Read the model definition and answer for the solid it produces. Units are mm, in the model's axes. Face numbers are marked on the shaded views. A direction names the side the tool comes from. Give positions to 0.01 mm unless a question says otherwise; leave off trailing zeros. Order: outer loops, then holes, each group sorted by start corner. A loop starts at its lowest first (then second) coordinate and runs counter-clockwise, first axis right, second up. Notation, with made-up numbers: (0.25, 43) -> (35.25, 43) arc R17 ccw to (35.25, 55) -> close; hole circle Ø7 at (79.25, 52). An arc over 180 degrees is marked (long way). One line per question, with ' | ' between items. Start each with the question number.
```python
from build123d import *

# Parameters (mm, degrees)
BASE_FLANGE1_DEPTH = 52
CUT_EXTRUDE1_DEPTH = 88.177978871
FILLET1_R          = 2
SKETCH7_R          = 12
SKETCH7_R_2        = 1.75
CUT_EXTRUDE2_DEPTH = 10
SKETCH8_R          = 2.8
CUT_EXTRUDE3_DEPTH = 2
SKETCH9_W          = 8
SKETCH9_H          = 10
CUT_EXTRUDE4_DEPTH = 10
SKETCH10_R         = 2.1
CUT_EXTRUDE5_DEPTH = 10


# Sheet-metal steps are written as plain solids
with BuildPart() as part:
    # Sketch1 → Base-Flange1 (new body)
    with BuildSketch(Plane(origin=(0, 0, 0), x_dir=(1, 0, 0), z_dir=(0, 1, 0))):
        with BuildLine():
            Line((36, 0), (2.8, 0))
            ThreePointArc((2.8, 0), (0.820101013, 0.820101013), (0, 2.8))
            Line((0, 2.8), (0, 60))
            Line((0, 60), (2, 60))
            Line((2, 60), (2, 2.8))
            ThreePointArc((2, 2.8), (2.234314575, 2.234314575), (2.8, 2))
            Line((2.8, 2), (36, 2))
            Line((36, 2), (36, 0))
        make_face()
    extrude(amount=BASE_FLANGE1_DEPTH)

    # Sketch6 → Cut-Extrude1 (cut, through all)
    with BuildSketch(Plane.ZY):
        Polygon((-18.8, 52), (-2.8, 36), (0, 36), (0, 52), align=None)
        Polygon((-60, 52), (-58.585786438, 52), (-60, 50.585786438), align=None)
        Polygon((-60, 1.414213562), (-60, 0), (-58.585786438, 0), align=None)
    extrude(amount=-CUT_EXTRUDE1_DEPTH, mode=Mode.SUBTRACT)

    # Fillet1
    fillet1_edges = [part.edges().sort_by_distance(p)[0] for p in [
        (36, 36, -1),
        (36, 0, -1),
    ]]
    fillet(fillet1_edges, radius=FILLET1_R)

    # Sketch7 → Cut-Extrude2 (cut)
    with BuildSketch(Plane(origin=(2, 0, 0), x_dir=(0, 0, -1), z_dir=(1, 0, 0))):
        with Locations((39, 31)):
            Circle(SKETCH7_R)
        with Locations((54.5, 46.5)):
            Circle(SKETCH7_R_2)
        with Locations(Location((23.5, 46.5, 0), (0, 0, 180))):
            Circle(SKETCH7_R_2)
        with Locations(Location((54.5, 15.5, 0), (0, 0, 180))):
            Circle(SKETCH7_R_2)
        with Locations((23.5, 15.5)):
            Circle(SKETCH7_R_2)
    extrude(amount=-CUT_EXTRUDE2_DEPTH, mode=Mode.SUBTRACT)

    # Sketch8 → Cut-Extrude3 (cut)
    with BuildSketch(Plane.XY):
        with Locations((28, 29)):
            Circle(SKETCH8_R)
        with Locations(Location((28, 9, 0), (0, 0, 180))):
            Circle(SKETCH8_R)
        with Locations((8, 9)):
            Circle(SKETCH8_R)
        with Locations(Location((8, 29, 0), (0, 0, 180))):
            Circle(SKETCH8_R)
    extrude(amount=-CUT_EXTRUDE3_DEPTH, mode=Mode.SUBTRACT)

    # Sketch9 → Cut-Extrude4 (cut)
    with BuildSketch(Plane(origin=(0, 0, -2), x_dir=(-1, 0, 0), z_dir=(0, 0, -1))):
        with Locations((-18, 27)):
            Rectangle(SKETCH9_W, SKETCH9_H)
    extrude(amount=-CUT_EXTRUDE4_DEPTH, mode=Mode.SUBTRACT)

    # Sketch10 → Cut-Extrude5 (cut)
    with BuildSketch(Plane(origin=(2, 0, 0), x_dir=(0, 0, -1), z_dir=(1, 0, 0))):
        with Locations((15, 34)):
            Circle(SKETCH10_R)
    extrude(amount=-CUT_EXTRUDE5_DEPTH, mode=Mode.SUBTRACT)


solid = part.part
```
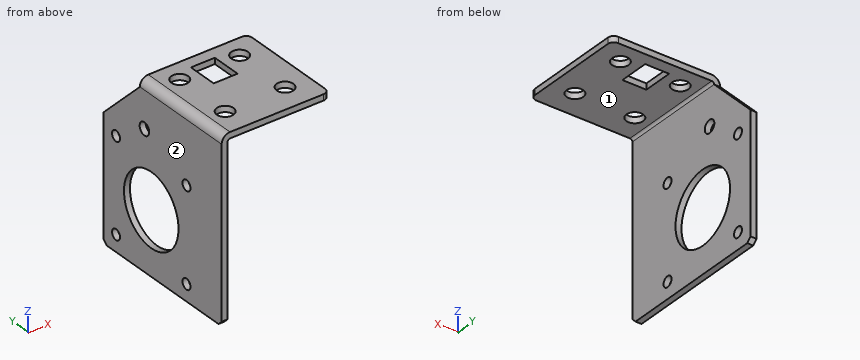
Q1. A cutting plane is placed at A-A, the plane z = -15. Determine the outline of the cut face in (x, y), then the cut area to 3 significant figures.
Q2. Find the intervals of material crossed by line 1 (Y direction, x = 8, z = -1.3); line 2 (Y direction, x = 1.15, z = -23.5); line 3 (Z direction, x = 1, y = 15), in increasing order.
Q3. A cutting plane is placed at C-C, the plane z = -23.5. Determine the outline of the cut face in (x, y), then the cut area to 3 significant figures.
Q4. A cutting plane is placed at D-D, the plane y = 5. Determine the outline of the cut face in (x, z).
Q5. Given P1, Ø5.5, axis at y = 15.5, z = -23.5, coming from the +X side; P2, Ø5, axis at x = 11.5, y = 10.5, coming from the -Z side; P3, Ø3, axis at x = 19.5, z = -1.5, coming from the +Y side, each flat-ended and moving along its own axis, determine where each tip first touches the part or whether it passes through.
Q6. A cutting plane is placed at B-B, the plane y = 46.5. Determine the outline of the cut face in (x, z).
Q7. Which of the six approach directions +Z, -Z, +X, -X, +Y, -Y give full straight-line access (tool end or side, diameter ignored) to the marked faces 1 and 2?
Geometry results:
1) outline: (0, 0) -> (2, 0) -> (2, 31.9) -> (0, 31.9) -> close; (0, 36.1) -> (2, 36.1) -> (2, 48.2) -> (0, 48.2) -> close | area: 88.0 mm²
2) line 1: 0 to 6.2, 11.8 to 26.2, 31.8 to 36 | line 2: 0 to 13.75, 17.25 to 44.75, 48.25 to 52 | line 3: -60 to -56.18, -52.82 to -25.18, -21.82 to -0.66
3) outline: (0, 0) -> (2, 0) -> (2, 13.75) -> (0, 13.75) -> close; (0, 17.25) -> (2, 17.25) -> (2, 44.75) -> (0, 44.75) -> close; (0, 48.25) -> (2, 48.25) -> (2, 52) -> (0, 52) -> close | area: 90.0 mm²
4) outline: (0, -60) -> (2, -60) -> (2, -2.8) arc R0.8 cw to (2.8, -2) -> (36, -2) -> (36, 0) -> (2.8, 0) arc R2.8 ccw to (0, -2.8) -> close
5) P1: x = 2 | P2: z = -2 | P3: y = 36
6) outline: (0, -60) -> (2, -60) -> (2, -56.25) -> (0, -56.25) -> close; (0, -52.75) -> (2, -52.75) -> (2, -25.25) -> (0, -25.25) -> close; (0, -21.75) -> (2, -21.75) -> (2, -13.3) -> (0, -13.3) -> close
7) face 1: -Z, +X, +Y, -Y | face 2: +Z, -Z, -X, +Y, -Y
